Geometry check sheet. Reference: the model listing, model coordinates, mm. A direction names the side the tool comes from. Coordinates: 2 decimals unless noted, no trailing zeros. Loops run counter-clockwise (first coordinate to the right, second up) from the corner with the lowest first, then second, coordinate; pieces in that order, holes last. Notation, with made-up numbers: M 31.5,62.5 L 49.5,62.5 A17 ccw 49.5,70.5 Z; hole C 12.5,-17 d10. An arc over 180 degrees is marked long. One line per question, with ' | ' between items. Start each with the question number.
from build123d import *

# Parameters (mm, degrees)
SKETCH048_R          = 23.6
PAD003_DEPTH         = 1.6
SKETCH049_R          = 23.6
PAD004_DEPTH         = 5
SKETCH050_R          = 26.5
SKETCH050_R_2        = 23.6
PAD005_DEPTH         = 1
SKETCH051_R          = 33.6
SKETCH051_R_2        = 13.875
PAD006_DEPTH         = 1.5
SKETCH052_R          = 1.6
POCKET001_DEPTH      = 7.501
POCKET001_DEPTH_BACK = 0.001


with BuildPart() as part:
    # Sketch048 → Pad003 (new body)
    with BuildSketch(Plane.XY):
        with BuildLine():
            ThreePointArc((11.420042, 23.942616), (-3.232792, 26.328981), (-16.873061, 20.46866))
            Line((-16.873061, 20.46866), (-16.156387, 19.599264))
            ThreePointArc((-16.156387, 19.599264), (-24.016172, 8.269431), (-24.797919, -5.497566))
            Line((-25.897919, -5.74143), (-24.797919, -5.497566))
            ThreePointArc((-25.897919, -5.74143), (-20.320637, -17.051039), (-10.151331, -24.507482))
            Line((-10.151331, -24.507482), (-9.720159, -23.46654))
            ThreePointArc((-9.720159, -23.46654), (2.765219, -25.249031), (14.568841, -20.806462))
            Line((15.215094, -21.729407), (14.568841, -20.806462))
            ThreePointArc((15.215094, -21.729407), (23.529477, -12.24867), (26.526707, 0))
            Line((26.526707, 0), (25.4, 0))
            ThreePointArc((25.4, 0), (21.481487, 13.553809), (10.934982, 22.925666))
            Line((11.420042, 23.942616), (10.934982, 22.925666))
        make_face()
        Circle(SKETCH048_R, mode=Mode.SUBTRACT)
    extrude(amount=-PAD003_DEPTH)

    # Sketch049 → Pad004 (join)
    with BuildSketch(Plane.XY):
        with BuildLine():
            ThreePointArc((11.324142, 23.958585), (10.481101, 24.339197), (9.62529, 24.690156))
            Line((9.62529, 24.690156), (9.2003, 23.6))
            ThreePointArc((9.2003, 23.6), (-10.018324, -23.264538), (10.824142, 22.900731))
            Line((11.324142, 23.958585), (10.824142, 22.900731))
        make_face()
        Circle(SKETCH049_R, mode=Mode.SUBTRACT)
    extrude(amount=-PAD004_DEPTH)

    # Sketch050 (on DatumPlane) → Pad005 (join)
    with BuildSketch(Plane.XY.offset(-5)):
        Circle(SKETCH050_R)
        Circle(SKETCH050_R_2, mode=Mode.SUBTRACT)
    extrude(amount=-PAD005_DEPTH)

    # Sketch051 (on DatumPlane) → Pad006 (join)
    with BuildSketch(Plane.XY.offset(-6)):
        Circle(SKETCH051_R)
        Circle(SKETCH051_R_2, mode=Mode.SUBTRACT)
    extrude(amount=-PAD006_DEPTH)

    # Sketch052 → Pocket001 (cut, two sides)
    with BuildSketch(Plane.XY) as pocket001_sk:
        with Locations((20.9, 20.9)):
            Circle(SKETCH052_R)
    extrude(amount=-POCKET001_DEPTH, mode=Mode.SUBTRACT)
    extrude(pocket001_sk.sketch, amount=POCKET001_DEPTH_BACK, mode=Mode.SUBTRACT)


with BuildPart() as part_1:
    # Body010 placement: moved
    add(part.part.moved(Location((0, -230, 0))))


solid = part_1.part
1. Draft check along Y on faces 1 (the cylindrical face through (2.588, -255.268, -0.789)), 2 (the flat face through (0, -206, 0)), 3 (the flat face through (10, -240, -6)). Enter one of: +Y half, -Y half, draft (parallel to the pull), parting line (faces both ways), or undercut.
2. Tool access check on faces 4 (the flat face through (25.4, -233.2, -1.6)), 5 (the cylindrical face through (-3.024, -203.646, -0.789)), 6 (the cylindrical face through (-20.435, -246.914, -0.789)). Record the directions out of +Z, -Z, +X, -X, +Y, -Y that give a thin tool (end or side, any length) a straight path to the whole face; none if there is none.
3. Sectioned sample at B-B (z = -2.75). Record the cut outline in (x, y).
4. Sectioned sample at C-C (x = 7.5). Record the cut outline in (y, z), and give its area (3 significant figures).
5. Sectioned sample at A-A (x = 0). Record the cut outline in (y, z) (3 decimals), and give its area (3 significant figures).
6. Depth check by flat-ended pin: pin 1 Ø4 at (y, z) = (-225.5, -2) entering from -X; pin 2 Ø1 at (y, z) = (-230, -1) entering from +X; pin 3 Ø23.5 at (x, y) = (-6, -233.5) entering from +Z; pin 4 Ø2.5 at (x, y) = (20.9, -209.1) entering from -Z. Enter the tip coordinate at first touch or a pass-through.
7. Thickness scan on line 1 (Y direction, x = 0, z = -4.8); line 2 (Z direction, x = 18, y = -242); line 3 (Y direction, x = -10.5, z = -1.5). Record the ranges inside material, lowest first.
Result:
1) face 1: -Y half | face 2: draft | face 3: undercut
2) face 4: none | face 5: +Z, +Y | face 6: +Z, -X, -Y
3) outline: M 9.2,-206.4 A25.33 ccw long 10.82,-207.1 L 11.32,-206.04 A26.5 ccw 9.63,-205.31 Z; hole C 0,-230 d47.2
4) outline: M -262.75,-7.5 L -241.67,-7.5 L -241.67,-6 L -252.38,-6 L -252.38,0 L -254.27,0 L -254.27,-1.6 L -254.19,-1.6 L -254.19,-5 L -255.42,-5 L -255.42,-6 L -262.75,-6 Z; M -218.33,-7.5 L -197.25,-7.5 L -197.25,-6 L -204.58,-6 L -204.58,-5 L -205.81,-5 L -205.81,-1.6 L -204.56,-1.6 L -204.56,0 L -207.62,0 L -207.62,-6 L -218.33,-6 Z | area: 89.6 mm2
5) outline: M -263.6,-7.5 L -243.875,-7.5 L -243.875,-6 L -253.6,-6 L -253.6,0 L -255.4,0 L -255.4,-1.6 L -255.33,-1.6 L -255.33,-5 L -256.5,-5 L -256.5,-6 L -263.6,-6 Z; M -216.125,-7.5 L -196.4,-7.5 L -196.4,-6 L -203.5,-6 L -203.5,-5 L -204.67,-5 L -204.67,-1.6 L -203.473,-1.6 L -203.473,0 L -206.4,0 L -206.4,-6 L -216.125,-6 Z | area: 84.3 mm2
6) pin 1: stops at x = -25.27 | pin 2: stops at x = 26.53 | pin 3: stops at z = -6 | pin 4: passes through
7) line 1: y = -255.33 to -253.6, -206.4 to -204.67 | line 2: z = -7.5 to -6 | line 3: y = -254.36 to -251.14, -208.86 to -205.64
